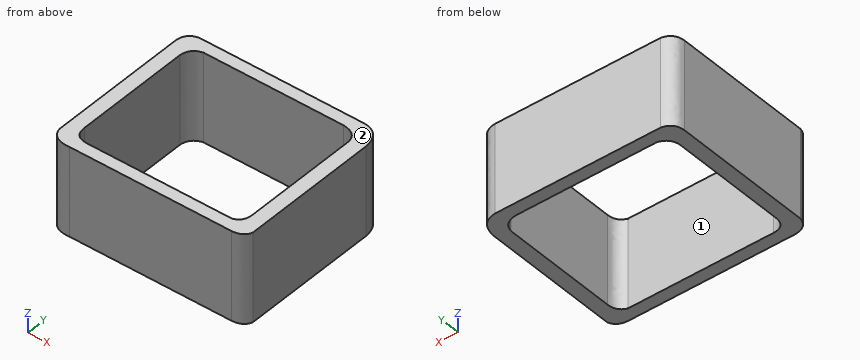
from build123d import *

# Parameters (mm, degrees)
BOSS_EXTRUDE4_DEPTH = 16


with BuildPart() as part:
    # Sketch3 → Boss-Extrude4 (new body)
    with BuildSketch(Plane.XY):
        with BuildLine():
            Line((-15.394959284, 15), (14.37206817, 15))
            add(Edge.make_bspline(
                [(14.37206817, 15), (16.344314338, 14.806153618), (17.421724303, 13.573948287), (17.604298066, 11.303384007)],
                knots=[0.157316623, 0.157316623, 0.157316623, 0.157316623, 1, 1, 1, 1], degree=3))
            Line((17.604298066, 11.303384007), (17.604298066, -13.324081778))
            add(Edge.make_bspline(
                [(17.604298066, -13.324081778), (17.337095636, -14.377577199), (16.496568016, -14.936216606), (15.082715206, -15)],
                knots=[0.317898453, 0.317898453, 0.317898453, 0.317898453, 1, 1, 1, 1], degree=3))
            Line((15.082715206, -15), (-13.989571853, -15))
            add(Edge.make_bspline(
                [(-17.604298066, -12.776063834), (-17.290256291, -14.390282227), (-16.085347553, -15.131594282), (-13.989571853, -15)],
                knots=[0.26063532, 0.26063532, 0.26063532, 0.26063532, 1, 1, 1, 1], degree=3))
            Line((-17.604298066, -12.776063834), (-17.604298066, 12.407487922))
            add(Edge.make_bspline(
                [(-17.604298066, 12.407487922), (-17.542065798, 14.610208227), (-15.394959284, 15)],
                knots=[0, 0, 0, 1, 1, 1], degree=2))
        make_face()
        with BuildLine():
            Line((-12.868921273, 12.851448393), (12.290353953, 12.851448393))
            add(Edge.make_bspline(
                [(12.290353953, 12.851448393), (13.937663202, 12.716565565), (14.868450289, 11.970465373), (15.082715212, 10.613147816)],
                knots=[0, 0, 0, 0, 0.769802432, 0.769802432, 0.769802432, 0.769802432], degree=3))
            Line((15.082715212, 10.613147816), (15.082715212, -10.422758289))
            add(Edge.make_bspline(
                [(15.082715212, -10.422758289), (15.08124759, -12.316637726), (13.415493999, -12.851448393)],
                knots=[0, 0, 0, 1, 1, 1], degree=2))
            Line((13.415493999, -12.851448393), (-12.720345322, -12.851448393))
            add(Edge.make_bspline(
                [(-15.082715206, -10.422758289), (-15.079137607, -12.799186037), (-12.720345322, -12.851448393)],
                knots=[0, 0, 0, 1, 1, 1], degree=2))
            Line((-15.082715206, -10.422758289), (-15.082715206, 10.375039522))
            add(Edge.make_bspline(
                [(-15.082715206, 10.375039522), (-14.901913362, 12.422179601), (-12.868921273, 12.851448393)],
                knots=[0, 0, 0, 1, 1, 1], degree=2))
        make_face(mode=Mode.SUBTRACT)
    extrude(amount=BOSS_EXTRUDE4_DEPTH)


solid = part.part
The listing builds one solid part. Answer for the finished solid, in the listing's coordinates (mm). Face numbers are marked on the shaded views. A direction names the side the tool comes from. Round coordinates to 2 decimals unless told otherwise and drop trailing zeros. Order: outer loops, then holes, each group sorted by start corner. A loop starts at its lowest first (then second) coordinate and runs counter-clockwise, first axis right, second up. Notation, with made-up numbers: M 83.5,-5 L 91.5,-5 A15 cw 91.5,1 Z; hole C 15.25,70.25 d2. An arc over 180 degrees is marked long. Answer in a Markdown table with one row per item. Add a question column.
1) The part is cut by section A-A on x = -4.5. Determine the outline of the cut face in (y, z).
2) Consider line 1 along X through (y, z) = (-10, 1.5); line 2 along Y through (x, z) = (11.5, 10.5); line 3 along Y through (x, z) = (-14.5, 3.5). Determine where each line is inside the solid, lowest interval first. Write a range as from..to.
3) The part is cut by section B-B on y = -0.5. Determine the outline of the cut face in (x, z), plus the area to 3 significant figures.
4) Which of the six approach directions +Z, -Z, +X, -X, +Y, -Y give full straight-line access (tool end or side, diameter ignored) to the marked faces 1 and 2?
5) A flat-ended cylindrical pin translates along its axis: pin 1 Ø8 at (x, z) = (6, 7) entering from -Y. Find the tip coordinate at first contact, or state that the pin passes through.
Findings below:
| question | item | result |
|---|---|---|
| 1 | outline | M -15,0 L -12.85,0 L -12.85,16 L -15,16 Z; M 12.85,0 L 15,0 L 15,16 L 12.85,16 Z |
| 2 | line 1 | x = -17.6..-15.08, 15.08..17.6 |
| 2 | line 2 | y = -15..-12.85, 12.85..15 |
| 2 | line 3 | y = -15.01..-12.21, 11.95..15 |
| 3 | outline | M -17.6,0 L -15.08,0 L -15.08,16 L -17.6,16 Z; M 15.08,0 L 17.6,0 L 17.6,16 L 15.08,16 Z |
| 3 | area | 80.7 mm² |
| 4 | face 1 | +Z, -Z |
| 4 | face 2 | +Z, +X, -X, +Y, -Y |
| 5 | pin 1 | stops at y = -15 |
